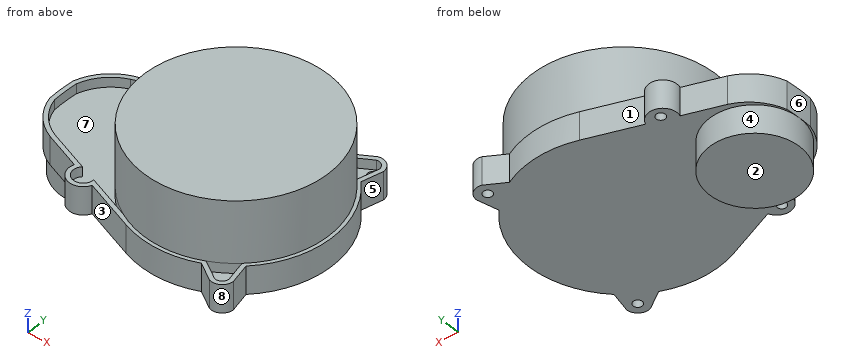
```python
from build123d import *

# Parameters (mm, degrees)
ESQUISSE1_R             = 1.6
BOSS_EXTRU_1_DEPTH      = 10
ESQUISSE2_R             = 32.8
BOSS_EXTRU_2_DEPTH      = 22
ENL_V_MAT_EXTRU_1_DEPTH = 3.5
BOSS_EXTRU_3_REACH      = 12
ESQUISSE5_R             = 16
BOSS_EXTRU_4_DEPTH      = 10


with BuildPart() as part:
    # Esquisse1 → Boss.-Extru.1 (new body)
    with BuildSketch(Plane.XY):
        with BuildLine():
            ThreePointArc((-52.114163482, -17.022112424), (-58.887228209, -12.14530881), (-62.818181851, -4.782889184))
            ThreePointArc((-62.818181851, -4.782889184), (-63, 0), (-62.818181851, 4.782889184))
            ThreePointArc((-62.818181851, 4.782889184), (-58.887228209, 12.14530881), (-52.114163482, 17.022112424))
            Line((-52.114163482, 17.022112424), (-39.149984877, 21.802247897))
            ThreePointArc((-39.149984877, 21.802247897), (-36.188478781, 28.223266636), (-29.767460042, 25.26176054))
            Line((-29.767460042, 25.26176054), (-11.762342986, 31.900584438))
            ThreePointArc((-11.762342986, 31.900584438), (1.39665257, 33.97130203), (14.341260705, 30.827394333))
            Line((14.341260705, 30.827394333), (20.756023105, 34.801647207))
            ThreePointArc((20.756023105, 34.801647207), (24.347774736, 34.238511045), (26, 31))
            Line((26, 31), (24.288429708, 23.792271483))
            ThreePointArc((24.288429708, 23.792271483), (34, 0), (24.288429708, -23.792271483))
            Line((24.288429708, -23.792271483), (26, -31))
            ThreePointArc((26, -31), (24.347774736, -34.238511045), (20.756023105, -34.801647207))
            Line((20.756023105, -34.801647207), (14.341260705, -30.827394333))
            ThreePointArc((14.341260705, -30.827394333), (1.39665257, -33.97130203), (-11.762342986, -31.900584438))
            Line((-11.762342986, -31.900584438), (-29.767460042, -25.26176054))
            ThreePointArc((-29.767460042, -25.26176054), (-36.188478781, -28.223266636), (-39.149984877, -21.802247897))
            Line((-39.149984877, -21.802247897), (-52.114163482, -17.022112424))
        make_face()
        with Locations((-35, -25)):
            Circle(ESQUISSE1_R, mode=Mode.SUBTRACT)
        with Locations((22, 31)):
            Circle(ESQUISSE1_R, mode=Mode.SUBTRACT)
        with Locations((-35, 25)):
            Circle(ESQUISSE1_R, mode=Mode.SUBTRACT)
        with Locations((22, -31)):
            Circle(ESQUISSE1_R, mode=Mode.SUBTRACT)
    extrude(amount=BOSS_EXTRU_1_DEPTH)

    # Esquisse2 → Boss.-Extru.2 (add)
    with BuildSketch(Plane.XY.offset(10)):
        Circle(ESQUISSE2_R)
    extrude(amount=BOSS_EXTRU_2_DEPTH)

    # Esquisse3 → Enlèv. mat.-Extru.1 (cut)
    with BuildSketch(Plane.XY.offset(10)):
        with BuildLine():
            Line((-51.564604514, -15.626028317), (-36.906810431, -21.030631539))
            ThreePointArc((-36.906810431, -21.030631539), (-35.669551885, -26.815887911), (-30.972780695, -23.218619448))
            Line((-30.972780695, -23.218619448), (-11.24341609, -30.493205713))
            ThreePointArc((-11.24341609, -30.493205713), (1.736287169, -32.453586965), (14.43273391, -29.119515653))
            Line((14.43273391, -29.119515653), (21.375089208, -33.420637623))
            ThreePointArc((21.375089208, -33.420637623), (23.468804453, -33.02302088), (24.495170617, -31.155317718))
            Line((24.495170617, -31.155317718), (22.63500045, -23.321808563))
            ThreePointArc((22.63500045, -23.321808563), (32.5, 0), (22.63500045, 23.321808563))
            Line((22.63500045, 23.321808563), (24.495170617, 31.155317718))
            ThreePointArc((24.495170617, 31.155317718), (23.468804453, 33.02302088), (21.375089208, 33.420637623))
            Line((21.375089208, 33.420637623), (14.43273391, 29.119515653))
            ThreePointArc((14.43273391, 29.119515653), (1.736287169, 32.453586965), (-11.24341609, 30.493205713))
            Line((-11.24341609, 30.493205713), (-30.972780695, 23.218619448))
            ThreePointArc((-30.972780695, 23.218619448), (-35.669551885, 26.815887911), (-36.906810431, 21.030631539))
            Line((-36.906810431, 21.030631539), (-51.564604514, 15.626028317))
            ThreePointArc((-51.564604514, 15.626028317), (-57.722932582, 11.197936413), (-61.33314674, 4.527152633))
            ThreePointArc((-61.33314674, 4.527152633), (-61.5, 0), (-61.33314674, -4.527152633))
            ThreePointArc((-61.33314674, -4.527152633), (-57.722932582, -11.197936413), (-51.564604514, -15.626028317))
        make_face()
    extrude(amount=-ENL_V_MAT_EXTRU_1_DEPTH, mode=Mode.SUBTRACT)

    # Esquisse4 → Boss.-Extru.3 (add, up to next)
    with BuildSketch(Plane(origin=(0, 0, 10), x_dir=(-1, 0, 0), z_dir=(0, 0, -1)), mode=Mode.PRIVATE) as boss_extru_3_sk1:
        with BuildLine():
            Line((-22.715550233, 23.661018101), (-22.63500045, 23.321808563))
            ThreePointArc((-22.63500045, 23.321808563), (-32.5, 0), (-22.63500045, -23.321808563))
            Line((-22.63500045, -23.321808563), (-22.715550233, -23.661018101))
            ThreePointArc((-22.715550233, -23.661018101), (-18.935479047, -26.78222607), (-14.732448894, -29.305203456))
            Line((-14.732448894, -29.305203456), (-14.43273391, -29.119515653))
            ThreePointArc((-14.43273391, -29.119515653), (-1.736287169, -32.453586965), (11.24341609, -30.493205713))
            Line((11.24341609, -30.493205713), (15.396177122, -28.962004938))
            ThreePointArc((15.396177122, -28.962004938), (32.8, 0), (15.396177122, 28.962004938))
            Line((15.396177122, 28.962004938), (11.24341609, 30.493205713))
            ThreePointArc((11.24341609, 30.493205713), (-1.736287169, 32.453586965), (-14.43273391, 29.119515653))
            Line((-14.43273391, 29.119515653), (-14.732448894, 29.305203456))
            ThreePointArc((-14.732448894, 29.305203456), (-18.935479047, 26.78222607), (-22.715550233, 23.661018101))
        make_face()
    boss_extru_3_tool1 = extrude(boss_extru_3_sk1.sketch, amount=BOSS_EXTRU_3_REACH, mode=Mode.PRIVATE) - part.part
    add(boss_extru_3_tool1.solids().sort_by_distance((-0.139045, 0, 10))[0])

    # Esquisse5 → Boss.-Extru.4 (add)
    with BuildSketch(Plane(origin=(0, 0, 0), x_dir=(-1, 0, 0), z_dir=(0, 0, -1))):
        with Locations((47, 0)):
            Circle(ESQUISSE5_R)
    extrude(amount=BOSS_EXTRU_4_DEPTH)


solid = part.part
```
Geometry: final body of the model. Coordinates: model frame, mm. Face numbers are marked on the shaded views. A direction names the side the tool comes from. Round coordinates to 2 decimals unless told otherwise and drop trailing zeros. Loops run counter-clockwise (first coordinate to the right, second up) from the corner with the lowest first, then second, coordinate; pieces in that order, holes last. Notation, with made-up numbers: (-25.75, 57) -> (6.25, 57) arc R34 cw to (6.25, 91) -> close; hole circle Ø10 at (51, -27). An arc over 180 degrees is marked (long way). Use one line per item in the form item = value. Start each with the question number.
1) Line query: L1, parallel to Y at x = 22, z = 2.5; L2, parallel to Y at x = -35, z = 2; L3, parallel to Z at x = -28, y = 20. Output: solid intervals per line, ascending.
2) First-contact query: P1, Ø10.5, axis at x = 17.5, y = 28, coming from the +Z side; P2, Ø8, axis at x = -13, y = -19, coming from the -Z side; P3, Ø10, axis at x = -7, z = 18.5, coming from the +Y side; P4, Ø5, axis at x = 22, y = -31, coming from the +Z side. Flat tips, straight axial feed; report the tip coordinate or a pass-through.
3) Access query for the marked faces 1, 2, 3 and 4. Directions: +Z, -Z, +X, -X, +Y, -Y. A direction counts if a zero-diameter tool reaches every point of the face in a straight line with its end or side. Return the directions, or none.
4) Draft query along Y for the marked faces 5, 6, 7 and 8. Return one class per face: released by +Y, released by -Y, zero draft, split by the parting line, or undercut.
5) Section D-D on z = -1.5. Output: boundary loops of the cut face in (x, y).
6) Section B-B on y = -7.5. Output: boundary loops of the cut face in (x, z).
7) Section C-C on x = -47. Output: boundary loops of the cut face in (y, z), then the cut area to 3 significant figures.
8) Section A-A on x = -35. Output: boundary loops of the cut face in (y, z), then the cut area to 3 significant figures.
Response:
q1.L1 = -35 to -32.6, -29.4 to 29.4, 32.6 to 35
q1.L2 = -28.5 to -26.6, -23.4 to 23.4, 26.6 to 28.5
q1.L3 = 0 to 6.5
q2.P1 = 32
q2.P2 = 0
q2.P3 = 32.74
q2.P4 = 10
q3.face_1 = +Z, -Z, +Y
q3.face_2 = -Z, +X, -X, +Y, -Y
q3.face_3 = +Z, -Z, -Y
q3.face_4 = -Z
q4.face_5 = undercut
q4.face_6 = split by the parting line
q4.face_7 = undercut
q4.face_8 = released by -Y
q5.outline = circle Ø32 at (-47, 0)
q6.outline = (-61.86, 0) -> (-61.13, 0) -> (-61.13, -10) -> (-32.87, -10) -> (-32.87, 0) -> (33.16, 0) -> (33.16, 10) -> (31.93, 10) -> (31.93, 32) -> (-31.93, 32) -> (-31.93, 6.5) -> (-60.2, 6.5) -> (-60.2, 10) -> (-61.86, 10) -> close
q7.outline = (-18.91, 0) -> (-16, 0) -> (-16, -10) -> (16, -10) -> (16, 0) -> (18.91, 0) -> (18.91, 10) -> (17.31, 10) -> (17.31, 6.5) -> (-17.31, 6.5) -> (-17.31, 10) -> (-18.91, 10) -> close
q7.area = 577 mm^2
q8.outline = (-28.5, 0) -> (-26.6, 0) -> (-26.6, 6.5) -> (-26.99, 6.5) -> (-26.99, 10) -> (-28.5, 10) -> close; (-23.4, 0) -> (-10.58, 0) -> (-10.58, -10) -> (10.58, -10) -> (10.58, 0) -> (23.4, 0) -> (23.4, 6.5) -> (-23.4, 6.5) -> close; (26.6, 0) -> (28.5, 0) -> (28.5, 10) -> (26.99, 10) -> (26.99, 6.5) -> (26.6, 6.5) -> close
q8.area = 551 mm^2
